Check sheet for the modelled part. Datum: model origin and axes. Units: mm. A direction names the side the tool comes from. Give positions to 0.01 mm unless a question says otherwise; leave off trailing zeros. Loops run counter-clockwise (first coordinate to the right, second up) from the corner with the lowest first, then second, coordinate; pieces in that order, holes last. Notation, with made-up numbers: (26, 29.5) - (30, 29.5) arc R31 ccw to (30, 65.5) - close; hole circle Ø8 at (56, 76.5). An arc over 180 degrees is marked (long way). Answer in a Markdown table with one row per item. Add a question column.
(1) Go/stop test with flat-tipped pins: P1, Ø6, axis at y = -3.5, z = 17, coming from the -X side; P2, Ø3, axis at x = 169.5, y = -8, coming from the -Z side; P3, Ø8, axis at y = 17.5, z = 22.5, coming from the -X side; P4, Ø7, axis at x = 172, z = 22, coming from the -Y side. Record where each tip stops, or that it passes through.
(2) Draft check along Y on faces 1 (the face through (168, -6, 10)), 2 (the face through (-6, 0, 11)), 3 (the face through (46.542, -0.44, 18.958)). Enter one of: released by +Y, released by -Y, zero draft, split by the parting line, or undercut.
(3) Thickness scan on L1, parallel to Y at x = 140, z = 26; L2, parallel to X at y = -0.5, z = 18.5 (3 decimals); L3, parallel to Z at x = 172, y = 8. Record the ranges inside material, lowest first.
(4) Sectioned sample at B-B on x = 131.5. Enter the section's corners in (y, z), then the cut area to 3 significant figures.
(5) Sectioned sample at D-D on z = 31.5. Enter the section's corners in (x, y).
(6) Sectioned sample at C-C on y = -17. Enter the section's corners in (x, z).
(7) Sectioned sample at A-A on z = 4. Enter the section's corners in (x, y).
(8) Set-up check for faces 4 (the face through (166, -1, 22)), 5 (the face through (175.5, 11, 24.5)), 6 (the face through (13, 20, 19)), 7 (the face through (32.546, -0.132, 10.846)): record each of +Z, -Z, +X, -X, +Y, -Y from which the full face is reachable in a straight line by a thin tool's end or side.
from build123d import *

# Parameters (mm, degrees)
SKICA2_R                 = 15
P_IDAT_VYSUNUT_M1_DEPTH  = 16
P_IDAT_VYSUNUT_M2_DEPTH  = 22
SKICA2_4_R               = 15
P_IDAT_VYSUNUT_M3_DEPTH  = 44
SKICA3_R                 = 4
P_IDAT_VYSUNUT_M4_DEPTH  = 11
SKICA4_W                 = 50
SKICA4_H                 = 2
ODEBRAT_VYSUNUT_M1_DEPTH = 191.832387188


with BuildPart() as part:
    # Skica2 → P_idat vysunut_m1 (new body)
    # profile 1 of 3: a face of its own
    with BuildSketch(Plane.XY):
        with BuildLine():
            Line((0, -20), (26.547310648, -20))
            ThreePointArc((26.547310648, -20), (46.547310648, 0), (26.547310648, 20))
            Line((26.547310648, 20), (0, 20))
            ThreePointArc((0, 20), (-20, 0), (0, -20))
        make_face()
        with BuildLine():
            ThreePointArc((26.547310648, -6), (32.547310648, 0), (26.547310648, 6))
            Line((26.547310648, 6), (0, 6))
            ThreePointArc((0, 6), (-6, 0), (0, -6))
            Line((0, -6), (26.547310648, -6))
        make_face(mode=Mode.SUBTRACT)
    # profile 2 of 3: a face of its own
    with BuildSketch(Plane.XY):
        with BuildLine():
            Line((138.21656051, 24.936305732), (0, 20))
            Line((0, 20), (26.547310648, 20))
            ThreePointArc((26.547310648, 20), (46.547310648, 0), (26.547310648, -20))
            Line((26.547310648, -20), (0, -20))
            Line((0, -20), (138.21656051, -24.936305732))
            ThreePointArc((138.21656051, -24.936305732), (115, 0), (138.21656051, 24.936305732))
        make_face()
    # profile 3 of 3: a face of its own
    with BuildSketch(Plane.XY):
        with BuildLine():
            Line((140, 25), (138.21656051, 24.936305732))
            ThreePointArc((138.21656051, 24.936305732), (115, 0), (138.21656051, -24.936305732))
            Line((138.21656051, -24.936305732), (140, -25))
            ThreePointArc((140, -25), (157.67766953, -17.67766953), (165, 0))
            ThreePointArc((165, 0), (157.67766953, 17.67766953), (140, 25))
        make_face()
        with Locations((140, 0)):
            Circle(SKICA2_R, mode=Mode.SUBTRACT)
    extrude(amount=P_IDAT_VYSUNUT_M1_DEPTH)

    # Skica2_3 → P_idat vysunut_m2 (add)
    with BuildSketch(Plane.XY):
        with BuildLine():
            Line((0, -20), (26.547310648, -20))
            ThreePointArc((26.547310648, -20), (46.547310648, 0), (26.547310648, 20))
            Line((26.547310648, 20), (0, 20))
            ThreePointArc((0, 20), (-20, 0), (0, -20))
        make_face()
        with BuildLine():
            ThreePointArc((26.547310648, -6), (32.547310648, 0), (26.547310648, 6))
            Line((26.547310648, 6), (0, 6))
            ThreePointArc((0, 6), (-6, 0), (0, -6))
            Line((0, -6), (26.547310648, -6))
        make_face(mode=Mode.SUBTRACT)
    extrude(amount=P_IDAT_VYSUNUT_M2_DEPTH)

    # Skica2_4 → P_idat vysunut_m3 (add)
    with BuildSketch(Plane.XY):
        with BuildLine():
            Line((140, 25), (138.21656051, 24.936305732))
            ThreePointArc((138.21656051, 24.936305732), (115, 0), (138.21656051, -24.936305732))
            Line((138.21656051, -24.936305732), (140, -25))
            ThreePointArc((140, -25), (157.67766953, -17.67766953), (165, 0))
            ThreePointArc((165, 0), (157.67766953, 17.67766953), (140, 25))
        make_face()
        with Locations((140, 0)):
            Circle(SKICA2_4_R, mode=Mode.SUBTRACT)
    extrude(amount=P_IDAT_VYSUNUT_M3_DEPTH)

    # Skica3 → P_idat vysunut_m4 (add, symmetric)
    with BuildSketch(Plane(origin=(0, 0, 0), x_dir=(1, 0, 0), z_dir=(0, 1, 0))):
        with BuildLine():
            Line((172, -10), (156.52015128, -10))
            Line((156.52015128, -10), (156.52015128, -34))
            Line((156.52015128, -34), (172, -34))
            ThreePointArc((172, -34), (184, -22), (172, -10))
        make_face()
        with Locations(Location((172, -22, 0), (0, 0, 270))):
            Circle(SKICA3_R, mode=Mode.SUBTRACT)
    extrude(amount=P_IDAT_VYSUNUT_M4_DEPTH, both=True)

    # Skica4 → Odebrat vysunut_m1 (cut, through all)
    with BuildSketch(Plane.XY.offset(44)):
        with Locations((165, 0)):
            Rectangle(SKICA4_W, SKICA4_H)
    extrude(amount=-ODEBRAT_VYSUNUT_M1_DEPTH, mode=Mode.SUBTRACT)


solid = part.part
Reply:
| question | item | result |
|---|---|---|
| 1 | P1 | x = -19.99 |
| 1 | P2 | z = 10 |
| 1 | P3 | x = -14.73 |
| 1 | P4 | through |
| 2 | face 1 | zero draft |
| 2 | face 2 | undercut |
| 2 | face 3 | split by the parting line |
| 3 | L1 | -25 to -15, 15 to 25 |
| 3 | L2 | -19.994 to -5.979, 32.526 to 46.541, 115.005 to 125.008 |
| 3 | L3 | 10 to 18, 26 to 34 |
| 4 | outline | (-24.7, 0) - (-12.36, 0) - (-12.36, 44) - (-23.51, 44) - (-23.51, 16) - (-24.7, 16) - close; (12.36, 0) - (24.7, 0) - (24.7, 16) - (23.51, 16) - (23.51, 44) - (12.36, 44) - close |
| 4 | area | 1,020 mm^2 |
| 5 | outline | (138.22, -24.94) - (140, -25) arc R25 ccw to (162.45, -11) - (179.33, -11) - (179.33, -1) - (154.97, -1) arc R15 cw (long way) to (154.97, 1) - (179.33, 1) - (179.33, 11) - (162.45, 11) arc R25 ccw to (140, 25) - (138.22, 24.94) arc R25 ccw to start |
| 6 | outline | (-10.54, 0) - (158.33, 0) - (158.33, 44) - (121.67, 44) - (121.67, 16) - (37.08, 16) - (37.08, 22) - (-10.54, 22) - close |
| 7 | outline | (0, -20) - (140, -25) arc R25 ccw to (164.98, -1) - (154.97, -1) arc R15 cw (long way) to (154.97, 1) - (164.98, 1) arc R25 ccw to (140, 25) - (0, 20) arc R20 ccw to start; hole (0, -6) - (26.55, -6) arc R6 ccw to (26.55, 6) - (0, 6) arc R6 ccw to start |
| 8 | face 4 | +Z, -Z, +X |
| 8 | face 5 | +Z, -Z, +X, +Y |
| 8 | face 6 | +Z, -X, +Y |
| 8 | face 7 | +Z, -Z |
